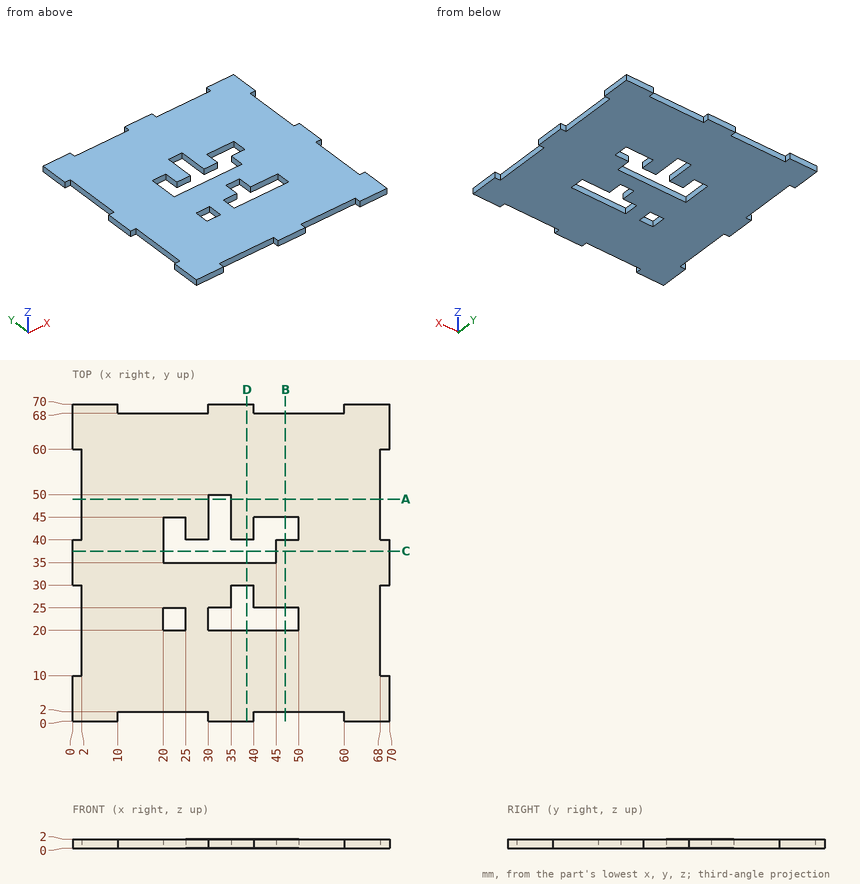
Geometry: see drawing. Coordinates: mm, zero at the bounding-box minimum. Round coordinates to 2 decimals unless told otherwise and drop trailing zeros. Loops run counter-clockwise (first coordinate to the right, second up) from the corner with the lowest first, then second, coordinate; pieces in that order, holes last.
(1) Material intervals for probe 1 along Y at (x, z) = (23, 1.35); probe 2 along Y at (x, z) = (39.5, 0.65); probe 3 along X at (y, z) = (25.5, 0.2), sorted ascending.
From the geometry:
probe 1: y = 2 to 20, 25 to 35, 45 to 68
probe 2: y = 0 to 20, 30 to 35, 40 to 70
probe 3: x = 2 to 35, 40 to 68
(2) Section query B-B (x = 47). Output: boundary loops of the cut face in (y, z), and give its area (3 significant figures).
From the geometry:
outline: (2, 0) - (20, 0) - (20, 2) - (2, 2) - close; (25, 0) - (40, 0) - (40, 2) - (25, 2) - close; (45, 0) - (68, 0) - (68, 2) - (45, 2) - close
area: 112 mm2
(3) Section query C-C (y = 37.5). Output: boundary loops of the cut face in (x, z), and give its area (3 significant figures).
From the geometry:
outline: (0, 0) - (20, 0) - (20, 2) - (0, 2) - close; (45, 0) - (70, 0) - (70, 2) - (45, 2) - close
area: 90.0 mm2
(4) Section query D-D (x = 38.5). Output: boundary loops of the cut face in (y, z).
From the geometry:
outline: (0, 0) - (20, 0) - (20, 2) - (0, 2) - close; (30, 0) - (35, 0) - (35, 2) - (30, 2) - close; (40, 0) - (70, 0) - (70, 2) - (40, 2) - close
(5) Section query A-A (y = 49). Output: boundary loops of the cut face in (x, z), and give its area (3 significant figures).
From the geometry:
outline: (2, 0) - (30, 0) - (30, 2) - (2, 2) - close; (35, 0) - (68, 0) - (68, 2) - (35, 2) - close
area: 122 mm2
